For this review, take the finished solid that the model builds, in its own axes (mm). A direction names the side the tool comes from. Give positions to 0.01 mm unless a question says otherwise; leave off trailing zeros. Order: outer loops, then holes, each group sorted by start corner. A loop starts at its lowest first (then second) coordinate and runs counter-clockwise, first axis right, second up. Notation, with made-up numbers: (8.5, 50) -> (59.5, 50) arc R38 cw to (59.5, 88) -> close; hole circle Ø2 at (-35.75, 65). An arc over 180 degrees is marked (long way). One line per item, written item: value. Start each with the question number.
from build123d import *

# Parameters (mm, degrees)
F0_W     = 10
F0_H     = 30
F0_R     = 17.5
F0_W_2   = 8
F0_H_2   = 15
F1_DEPTH = 15
F2_R     = 2


with BuildPart() as f1:
    # F0 (on Top) → F1 (new body)
    with BuildSketch(Plane.XY):
        with Locations((-82.245037, -15)):
            Rectangle(F0_W, F0_H)
        Polygon((-42.244907, -15), (-35.244778, 0), (-49.245037, 0), align=None)
        with BuildLine():
            Line((75.0551, 25), (-87.245037, 25))
            Line((-87.245037, 25), (-87.245037, 0))
            Line((-87.245037, 0), (-77.245037, 0))
            Line((-77.245037, 0), (-67.245037, 0))
            Line((-67.245037, 0), (-59.245037, 0))
            Line((-59.245037, 0), (-49.245037, 0))
            Line((-49.245037, 0), (-35.244778, 0))
            Line((-35.244778, 0), (75.0551, 0))
            ThreePointArc((75.0551, 0), (142.746842, 12.5), (75.0551, 25))
        make_face()
        with Locations((107.746842, 12.5)):
            Circle(F0_R, mode=Mode.SUBTRACT)
        with Locations((-63.245037, -7.5)):
            Rectangle(F0_W_2, F0_H_2)
    extrude(amount=F1_DEPTH)

    # F2
    f2_edges = [f1.edges().sort_by_distance(p)[0] for p in [
        (-87.245037, -2.5, 15),
        (-82.245037, -30, 15),
        (-77.245037, -15, 15),
        (-72.245037, 0, 15),
        (-67.245037, -7.5, 15),
        (-63.245037, -15, 15),
        (-59.245037, -7.5, 15),
        (-54.245037, 0, 15),
        (-45.744972, -7.5, 15),
        (-38.744843, -7.5, 15),
        (19.905161, 0, 15),
        (142.746842, 12.5, 15),
        (-6.094968, 25, 15),
        (90.246842, 12.5, 15),
        (19.905161, 0, 0),
        (75.0551, 0, 7.5),
        (75.0551, 25, 7.5),
        (142.746842, 12.5, 0),
        (-38.744843, -7.5, 0),
        (-45.744972, -7.5, 0),
        (-63.245037, -15, 0),
        (-82.245037, -30, 0),
        (-87.245037, 25, 7.5),
        (-6.094968, 25, 0),
        (-67.245037, -7.5, 0),
        (-87.245037, -2.5, 0),
        (90.246842, 12.5, 0),
    ]]
    fillet(f2_edges, radius=F2_R)


solid = f1.part
Q1. For line 1 along X through (y, z) = (-10, 6.25); line 2 along X through (y, z) = (-9.5, 14); line 3 along Y through (x, z) = (42, 2), list the stretches that pass through material, from the lowest coordinate up.
Q2. Take a section at A-A (z = 4.5). State the section outline as (x, y) points, and give its area (3 significant figures).
Q3. For pin 1 Ø4 at (y, z) = (-20, 11.5) entering from +X; pin 2 Ø4 at (x, z) = (-65, 5.5) entering from -Y; pin 3 Ø1.5 at (y, z) = (24, 7.5) entering from -X, all flat-tipped, find the tip position at first contact; note any pin that passes through.
Q4. Take a section at C-C (x = -16.5). State the section outline as (y, z) points, and give its area (3 significant figures).
Q5. Mouldability with a two-part tool opening along X and no side actions: class faces 1 (the flat face through (27, 14, 15)), 2 (the flat face through (-87.245, -3, 7)), 3 (the flat face through (-73, 0, 6)) as pulls with the +X half, pulls with the -X half, needs draft (parallel to the pull), parting line crosses it, or undercut.
Q6. Take a section at B-B (y = 12.5). State the section outline as (x, z) points, and give its area (3 significant figures).
Q7. For faces 4 (the cylindrical face through (-45.445, -6.795, 14.399)), 5 (the cylindrical face through (-45.18, -7.36, 0.6)), 6 (the cylindrical face through (103.953, -4.584, 7.423)), 7 (the flat face through (18, 0, 7)), 8 (the flat face through (-5, 25, 7)), list the 3-axis set-ups (+Z, -Z, +X, -X, +Y, -Y) from which the entire face can be reached by the end or side of a thin tool; tool diameter is ignored.
Answers below:
1. line 1: x = -87.25 to -77.25, -67.25 to -59.25, -44.58 to -39.91, 80.94 to 134.56
1. line 2: x = -86.98 to -77.51, -66.98 to -59.51, -44.52 to -39.97, 80.87 to 134.62
1. line 3: y = 0 to 25
2. outline: (-87.25, -30) -> (-77.25, -30) -> (-77.25, 0) -> (-67.25, 0) -> (-67.25, -15) -> (-59.25, -15) -> (-59.25, 0) -> (-49.25, 0) -> (-42.24, -15) -> (-35.24, 0) -> (73.71, 0) arc R2 cw to (75.55, -1.22) arc R35 ccw (long way) to (75.55, 26.22) arc R2 cw to (73.71, 25) -> (-85.25, 25) arc R2 ccw to (-87.25, 23) -> close; hole circle Ø35 at (107.75, 12.5)
2. area: 7,430 mm²
3. pin 1: stops at x = 124.92
3. pin 2: stops at y = -15
3. pin 3: stops at x = -87.23
4. outline: (0, 2) arc R2 ccw to (2, 0) -> (23, 0) arc R2 ccw to (25, 2) -> (25, 13) arc R2 ccw to (23, 15) -> (2, 15) arc R2 ccw to (0, 13) -> close
4. area: 372 mm²
5. face 1: needs draft
5. face 2: pulls with the -X half
5. face 3: undercut
6. outline: (-87.25, 2) arc R2 ccw to (-85.25, 0) -> (88.25, 0) arc R2 ccw to (90.25, 2) -> (90.25, 13) arc R2 ccw to (88.25, 15) -> (-85.25, 15) arc R2 ccw to (-87.25, 13) -> close; (125.25, 2) arc R2 ccw to (127.25, 0) -> (140.75, 0) arc R2 ccw to (142.75, 2) -> (142.75, 13) arc R2 ccw to (140.75, 15) -> (127.25, 15) arc R2 ccw to (125.25, 13) -> close
6. area: 2,920 mm²
7. face 4: +Z, -Y
7. face 5: -Z, -Y
7. face 6: +Z, -Z
7. face 7: +Z, -Z, -Y
7. face 8: +Z, -Z, -X, +Y
